Model file for the job. Use its own axes, mm. Face numbers are marked on the shaded views. Round coordinates to 2 decimals unless told otherwise and drop trailing zeros. Loops run counter-clockwise (first coordinate to the right, second up) from the corner with the lowest first, then second, coordinate; pieces in that order, holes last. Notation, with made-up numbers: (-17, -12.75) -> (-3, -12.75) arc R19 cw to (-3, 2.25) -> close; hole circle Ø1 at (86, -18). An arc over 180 degrees is marked (long way). Use a Markdown table: item, result. Add a question column.
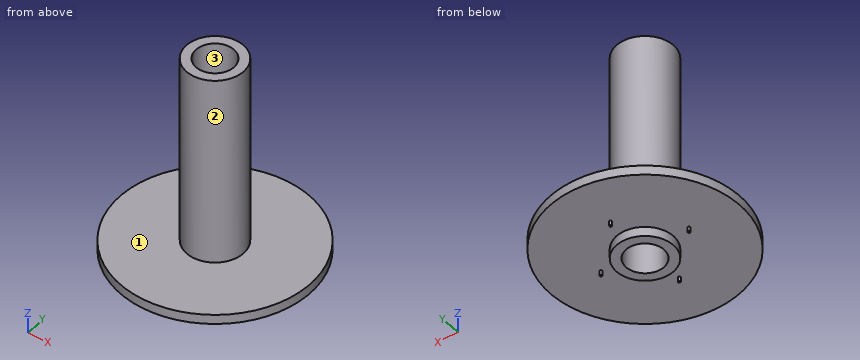
```python
from build123d import *

# Parameters (mm, degrees)
F0_R            = 63.5
F1_DEPTH        = 6.35
F2_R            = 0.7874
F3_DEPTH        = 3.175
F3_COPIES_COUNT = 4
F4_R            = 19.05
F5_DEPTH        = 6.35
F6_R            = 19.05
F7_DEPTH        = 127
F8_R            = 12.7
F9_DEPTH        = 139.701


# Not quite as in the source:
# - a pattern or mirror of a feature is missing from the dataset's text; its kind, count and spacing are read off the source's solid


with BuildPart() as f1:
    # F0 (on Top) → F1 (new body)
    with BuildSketch(Plane.XY):
        Circle(F0_R)
    extrude(amount=F1_DEPTH)

    # F2 (on face) → F3 (join)
    with BuildSketch(Plane(origin=(0, 0, 0), x_dir=(1, 0, 0), z_dir=(0, 0, -1))):
        with Locations((-30.1625, 0)):
            Circle(F2_R)
    f3 = extrude(amount=F3_DEPTH)

    # F3_copies: F3 ×4 about axis
    f3_copies_axis = Axis((0, 0, 0), (0, 0, 1))
    for i in range(1, F3_COPIES_COUNT):
        add(f3.rotate(f3_copies_axis, i * 360 / F3_COPIES_COUNT))

    # F4 (on face) → F5 (join)
    with BuildSketch(Plane(origin=(0, 0, 0), x_dir=(1, 0, 0), z_dir=(0, 0, -1))):
        Circle(F4_R)
    extrude(amount=F5_DEPTH)

    # F6 (on face) → F7 (join)
    with BuildSketch(Plane.XY.offset(6.35)):
        Circle(F6_R)
    extrude(amount=F7_DEPTH)

    # F8 (on face) → F9 (cut, through all)
    with BuildSketch(Plane.XY.offset(133.35)):
        Circle(F8_R)
    extrude(amount=-F9_DEPTH, mode=Mode.SUBTRACT)


solid = f1.part
```
1) Wall check: probe 1 along Y at (x, z) = (0, 74); probe 2 along Z at (x, y) = (-44.5, 10); probe 3 along X at (y, z) = (-3, 58.5). Give the ranges that are in metal, low to high. Write a range as from..to.
2) Pull direction Y, two halves, no side cores. Call the marked faces 1, 2 and 3: +Y half, -Y half, draft (parallel to the pull), parting line (faces both ways), or undercut.
3) Pin check, flat tips, straight feed: pin 1 Ø4 at (x, z) = (5.5, 13.5) entering from -Y; pin 2 Ø12 at (x, z) = (4.5, 32) entering from -Y; pin 3 Ø1.3 at (x, y) = (0, -30) entering from -Z (3 decimals); pin 4 Ø15 at (x, y) = (0, 0) entering from -Z. Stop position of each tip, or through.
4) Cut at C-C on y = 47. Write the cut outline in (x, z).
5) Cut at A-A on x = 10.5. Write the cut outline in (y, z), and give its area (3 significant figures).
6) Cut at B-B on z = 97. Write the cut outline in (x, y), and give its area (3 significant figures).
7) Cut at D-D on x = 36.5. Write the cut outline in (y, z), and give its area (3 significant figures).
Established:
| question | item | result |
|---|---|---|
| 1 | probe 1 | y = -19.05..-12.7, 12.7..19.05 |
| 1 | probe 2 | z = 0..6.35 |
| 1 | probe 3 | x = -18.81..-12.34, 12.34..18.81 |
| 2 | face 1 | draft |
| 2 | face 2 | parting line |
| 2 | face 3 | undercut |
| 3 | pin 1 | stops at y = -18.73 |
| 3 | pin 2 | stops at y = -19.05 |
| 3 | pin 3 | stops at z = -3.175 |
| 3 | pin 4 | passes through |
| 4 | outline | (-42.7, 0) -> (42.7, 0) -> (42.7, 6.35) -> (-42.7, 6.35) -> close |
| 5 | outline | (-62.63, 0) -> (-15.9, 0) -> (-15.9, -6.35) -> (-7.14, -6.35) -> (-7.14, 133.35) -> (-15.9, 133.35) -> (-15.9, 6.35) -> (-62.63, 6.35) -> close; (7.14, -6.35) -> (15.9, -6.35) -> (15.9, 0) -> (62.63, 0) -> (62.63, 6.35) -> (15.9, 6.35) -> (15.9, 133.35) -> (7.14, 133.35) -> close |
| 5 | area | 3,040 mm^2 |
| 6 | outline | circle Ø38.1 at (0, 0); hole circle Ø25.4 at (0, 0) |
| 6 | area | 633 mm^2 |
| 7 | outline | (-51.96, 0) -> (51.96, 0) -> (51.96, 6.35) -> (-51.96, 6.35) -> close |
| 7 | area | 660 mm^2 |
